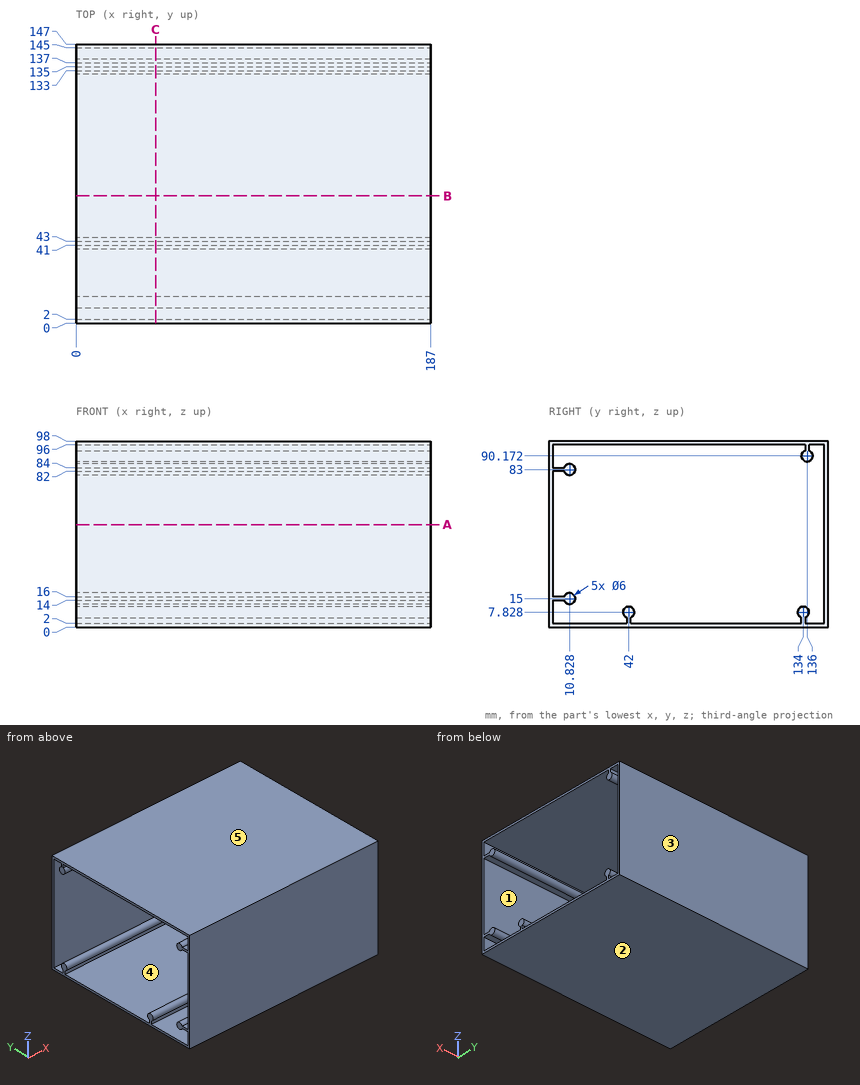
Design review of the part shown in the three views and the two pictorial views. Dimensions are in mm from the part's minimum x, y and z. A direction names the side the tool comes from. Give positions to 0.01 mm unless a question says otherwise; leave off trailing zeros. Loops run counter-clockwise (first coordinate to the right, second up) from the corner with the lowest first, then second, coordinate; pieces in that order, holes last. Notation, with made-up numbers: (-23.5, 36.5) - (-10.5, 36.5) arc R12 cw to (-10.5, 43.5) - close; hole circle Ø2 at (73, 85). An arc over 180 degrees is marked (long way). Write item = value, one per line.
1) Take a section at B-B on y = 67. State the section outline as (x, z) points.
Result sheet:
outline = (0, 0) - (187, 0) - (187, 2) - (0, 2) - close; (0, 96) - (187, 96) - (187, 98) - (0, 98) - close
2) Take a section at C-C on x = 42. State the section outline as (y, z) points, and give its area (3 significant figures).
Result sheet:
outline = (0, 0) - (147, 0) - (147, 98) - (0, 98) - close; hole (2, 2) - (41, 2) - (41, 5) arc R3 cw (long way) to (43, 5) - (43, 2) - (133, 2) - (133, 5) arc R3 cw (long way) to (135, 5) - (135, 2) - (145, 2) - (145, 96) - (137, 96) - (137, 93) arc R3 cw (long way) to (135, 93) - (135, 96) - (2, 96) - (2, 84) - (8, 84) arc R3 cw (long way) to (8, 82) - (2, 82) - (2, 16) - (8, 16) arc R3 cw (long way) to (8, 14) - (2, 14) - close
area = 1,150 mm2
3) Draft analysis for pull direction Y (two halves, no side actions). For the marked faces 1, 2 and 3, state which applies: +Y half, -Y half, draft (parallel to the pull), parting line (faces both ways), or undercut.
Result sheet:
face_1 = undercut
face_2 = draft
face_3 = +Y half
4) To check wall thickness, follow line 1 (Z direction, x = 143, y = 29); line 2 (Z direction, x = 160.5, y = 44) (1 decimal); line 3 (Y direction, x = 45.5, z = 24.5). State the ranges of each line that lie inside material, in increasing order.
Result sheet:
line_1 = 0 to 2, 96 to 98
line_2 = 0 to 2, 5.6 to 10.1, 96 to 98
line_3 = 0 to 2, 145 to 147
5) Take a section at A-A on z = 54. State the section outline as (x, y) points.
Result sheet:
outline = (0, 0) - (187, 0) - (187, 2) - (0, 2) - close; (0, 145) - (187, 145) - (187, 147) - (0, 147) - close
6) Tool access review of the marked faces 4 and 5: name each direction out of +Z, -Z, +X, -X, +Y, -Y from which nothing blocks a thin tool from reaching the whole face with its end or side.
Result sheet:
face_4 = +X, -X
face_5 = +Z, +X, -X, +Y, -Y
